Check sheet for the modelled part. Datum: model origin and axes. Units: mm. A direction names the side the tool comes from. Round coordinates to 2 decimals unless told otherwise and drop trailing zeros. Order: outer loops, then holes, each group sorted by start corner. A loop starts at its lowest first (then second) coordinate and runs counter-clockwise, first axis right, second up. Notation, with made-up numbers: M -26,-16 L -8,-16 A23 cw -8,-1 Z; hole C -2.75,13 d2. An arc over 180 degrees is marked long. One line per item, written item: value. Start each with the question number.
(1) Thickness scan on L1, parallel to Z at x = 6.25, y = 6; L2, parallel to X at y = 0.5, z = 3; L3, parallel to Y at x = 10.25, z = -5. Record the ranges inside material, lowest first.
(2) Access from +Z, -Z, +X, -X, +Y, -Y to the whole of each face (thin tool, end or side, straight path). Record for faces 1 (the face through (8, 4, 6)), 2 (the face through (8.1, 6.4, -0.1)), 3 (the face through (8, 4, -6)), 4 (the face through (1.93, 11.79, 11.75)).
(3) Release check for a two-part mould opening along X. For faces 5 (the face through (12.5, 4.46, 0.08)), 6 (the face through (8.285, 3.87, -4.337)), 7 (the face through (2, 0, -12.7)) record: released by +X, released by -X, zero draft, split by the parting line, or undercut.
(4) Cross-section at A-A, the plane z = 4. Enter the section's corners in (x, y), and give its area (3 significant figures).
(5) Cross-section at C-C, the plane z = 8. Enter the section's corners in (x, y), and give its area (3 significant figures).
(6) Cross-section at B-B, the plane y = 4.5. Count the separate pieces of the cut face and the enclosed holes in it, and give its area (3 significant figures).
(7) Depth check by flat-ended pin: pin 1 Ø3 at (x, y) = (5.5, 0) entering from -Z; pin 2 Ø4 at (y, z) = (7.5, -8.5) entering from +X; pin 3 Ø1 at (x, z) = (8.5, -4) entering from +Y. Enter the tip coordinate at first touch or a pass-through.
Autodesk Inventor part; units mm, degrees
ref_plane "Work Plane2" through (3.81, 12.7, -12.7) normal (0.9925462, 0.1218693, 0) x (0, 0, 1)
ref_plane "YZ Plane" through (0, 0, 0) normal (1, 0, 0) x (0, 1, 0)
ref_plane "XZ Plane" through (0, 0, 0) normal (0, 1, 0) x (-1, 0, 0)
sketch "Sketch1" plane through (0, 0, 0) normal (1, 0, 0) x (0, 1, 0)
  line L0 (-12.7, 12.7) -> (12.7, 12.7)
  line L1 (12.7, 12.7) -> (12.7, -12.7)
  line L2 (12.7, -12.7) -> (-12.7, -12.7)
  line L3 (-12.7, -12.7) -> (-12.7, 12.7)
  line L4 (-12.7, 12.7) -> (12.7, -12.7) construction
  line L5 (12.7, 12.7) -> (-12.7, -12.7) construction
  point P0 (0, 0)
  dimension "d0" = 25.4
  dimension "d1" = 25.4
extrude "Extrusion1" add sketch "Sketch1" along normal blind 3.81
ref_plane "Work Plane2" through (3.81, 12.7, -12.7) normal (0.9925462, 0.1218693, 0) x (0, 0, 1)
sketch "Sketch2" plane through (5.3342, 0.2862, 0) normal (0.9925462, 0.1218693, 0) x (0, 0, -1)
  line L0 (-6, 0.7324) -> (6, 0.7324)
  line L1 (6, 0.7324) -> (6, 5.7324)
  line L2 (6, 5.7324) -> (-6, 5.7324)
  line L3 (-6, 5.7324) -> (-6, 0.7324)
  line L4 (-6, 0.7324) -> (6, 5.7324) construction
  line L5 (6, 0.7324) -> (-6, 5.7324) construction
  point P0 (0, 0.366)
  point P1 (0, 3.2324)
  dimension "d4" = 12
  dimension "d5" = 5
extrude "Extrusion2" add sketch "Sketch2" along normal blind 7.62
sketch "Sketch3" plane through (3.81, 5.8744, 6) normal (-0.1218693, 0.9925462, 0) x (0.9925462, 0.1218693, 0)
  line L0 (8.4518, 12) -> (8.4518, 0)
  line L1 (13.7995, 6) -> (-14.4563, 6)
  point P0 (-4.4975, 6)
  point P1 (4.7518, 3)
  dimension "d8" = 3.7
  dimension "d9" = 3
hole "Hole1" at (8.5264, 6.4535, 3) direction (0.1218693, -0.9925462, 0) diameter 2.8956 end through all
mirror "Mirror1" about plane through (0, 0, 0) normal (0, 0, 1) of "Hole1"
sketch "Sketch4" plane through (0, 0, 0) normal (0, 0, 1) x (1, 0, 0)
  arc A0 (2.54, 0) -> (-200.66, 0) centre (-99.06, 0) ccw
  line L0 (0, 12.7) -> (0, -12.7)
  line L1 (-241.3, 0) -> (43.18, 0)
  line L2 (-200.66, 0) -> (2.54, 0)
  line L3 (-241.3, 0) -> (43.18, 0)
  point P0 (0, 0)
  dimension "d17" = 203.2
  dimension "d18" = 99.06
revolve "Revolution1" [suppressed]
fillet "Fillet1" radius 3.175 4 edges at (1.905, 12.7, -12.7) (1.905, 12.7, 12.7) (1.905, -12.7, 12.7) (1.905, -12.7, -12.7)
fillet "Fillet2" [suppressed]
sketch "Sketch5" plane through (5.3342, 0.2862, 0) normal (-0.9925462, -0.1218693, 0) x (0, 0, 1)
  line L0 (-6, 0.7324) -> (-6, 5.7324)
  line L1 (6, 0.7324) -> (-6, 0.7324)
  line L2 (6, 5.7324) -> (6, 0.7324)
  line L3 (-6, 5.7324) -> (6, 5.7324)
  point P0 (0, 0.366)
extrude "Extrusion3" add sketch "Sketch5" along normal up to surface surface through (3.81, 0, 0) normal (1, 0, 0)
ref_plane "Work Plane1" through (0, 0, 0) normal (0, 0, 1) x (1, 0, 0)
properties part number "BrakeShoeWithTilt_Base"
Values found:
1. L1: -6 to 6
1. L2: 0 to 3.81
1. L3: 1.63 to 6.67
2. face 1: +Z, +X, +Y, -Y
2. face 2: +Z, -Z, +Y
2. face 3: -Z, +X, +Y, -Y
2. face 4: +Z, +X, -X, +Y
3. face 5: released by +X
3. face 6: undercut
3. face 7: zero draft
4. outline: M 0,-12.7 L 3.81,-12.7 L 3.81,0.84 L 8.1,1.36 L 7.49,6.33 L 3.81,5.87 L 3.81,12.7 L 0,12.7 Z; M 9.57,6.58 L 10.17,1.62 L 12.81,1.94 L 12.2,6.9 Z
4. area: 130 mm^2
5. outline: M 0,-12.7 L 3.81,-12.7 L 3.81,12.7 L 0,12.7 Z
5. area: 96.8 mm^2
6. separate pieces: 1
6. enclosed holes: 2
6. area: 188 mm^2
7. pin 1: z = -6
7. pin 2: x = 3.81
7. pin 3: y = 6.48
